```python
from build123d import *

# Parameters (mm, degrees)
SKETCH1_R           = 6
SKETCH1_R_2         = 10
BOSS_EXTRUDE5_DEPTH = 5


with BuildPart() as part:
    # Sketch1 → Boss-Extrude5 (new body)
    with BuildSketch(Plane.XY):
        with BuildLine():
            ThreePointArc((-70.058465936, -58.078352807), (-72.989066837, -63.721836205), (-74, -70))
            Line((-74, -70), (-74, -102))
            ThreePointArc((-74, -102), (-57.94255977, -121.607555239), (-35.554377754, -109.730395847))
            ThreePointArc((-35.554377754, -109.730395847), (-10.665501502, -73.723982253), (26.649375188, -50.843467428))
            ThreePointArc((26.649375188, -50.843467428), (48.384433069, -44.417618227), (70.872883052, -47.241427079))
            ThreePointArc((70.872883052, -47.241427079), (100.915737424, -45.173387051), (91.224909648, -16.661323894))
            ThreePointArc((91.224909648, -16.661323894), (58.568789172, -9.425322294), (25.12069127, -9.506995785))
            ThreePointArc((25.12069127, -9.506995785), (17.4015399, -7.087809111), (13.997757222, 0.250584822))
            ThreePointArc((13.997757222, 0.250584822), (-3.45943961, 13.565849682), (-12.408356532, -6.483262156))
            ThreePointArc((-12.408356532, -6.483262156), (-11.834915893, -14.73854087), (-17.505199272, -20.765675115))
            ThreePointArc((-17.505199272, -20.765675115), (-45.782270653, -36.604484887), (-70.058465936, -58.078352807))
        make_face()
        with BuildLine():
            ThreePointArc((-44, -102), (-54, -112), (-64, -102))
            Line((-64, -102), (-64, -70))
            ThreePointArc((-64, -70), (-54, -60), (-44, -70))
            Line((-44, -70), (-44, -102))
        make_face(mode=Mode.SUBTRACT)
        Circle(SKETCH1_R, mode=Mode.SUBTRACT)
        with Locations((85.098500813, -34.646515436)):
            Circle(SKETCH1_R_2, mode=Mode.SUBTRACT)
    extrude(amount=BOSS_EXTRUDE5_DEPTH)


solid = part.part
```
Check sheet for the modelled part. Datum: model origin and axes. Units: mm. A direction names the side the tool comes from. Round coordinates to 2 decimals unless told otherwise and drop trailing zeros. Order: outer loops, then holes, each group sorted by start corner. A loop starts at its lowest first (then second) coordinate and runs counter-clockwise, first axis right, second up. Notation, with made-up numbers: (82, 18) - (136, 18) arc R22 ccw to (136, 30) - close; hole circle Ø11 at (53, -14). An arc over 180 degrees is marked (long way). Write item = value, one per line.
Q1. Thickness scan on line 1 along X through (y, z) = (-81, 3); line 2 along X through (y, z) = (-26, 1.4); line 3 along Y through (x, z) = (86.5, 0.45). Record the ranges inside material, lowest first.
Computed:
line_1 = -74 to -64, -44 to -17.65
line_2 = -28.51 to 80.07, 90.12 to 102.02
line_3 = -53.59 to -44.55, -24.75 to -15.14
Q2. Draft check along Y on faces 1 (the face through (-6, 0, 2)), 2 (the face through (-72.96, -63.64, 2.46)), 3 (the face through (100.641, -45.575, 2.465)). Enter one of: pulls with the +Y half, pulls with the -Y half, needs draft (parallel to the pull), parting line crosses it, or undercut.
Computed:
face_1 = undercut
face_2 = pulls with the +Y half
face_3 = parting line crosses it
Q3. Tool access check on faces 4 (the face through (-54, -60, 2)), 5 (the face through (1, -44, 5)). Record the directions out of +Z, -Z, +X, -X, +Y, -Y that give a thin tool (end or side, any length) a straight path to the whole face; none if there is none.
Computed:
face_4 = +Z, -Z
face_5 = +Z, +X, -X, +Y, -Y
Q4. Section check A-A (y = -97). Record the boundary of the cut face in (x, z).
Computed:
outline = (-74, 0) - (-64, 0) - (-64, 5) - (-74, 5) - close; (-44, 0) - (-29.18, 0) - (-29.18, 5) - (-44, 5) - close
Q5. Go/stop test with flat-tipped pins: pin 1 (2 mm diameter, centred on y = -33, z = 3.5, fed in from +X); pin 2 (1.5 mm diameter, centred on y = -79.5, z = 2.5, fed in from +X); pin 3 (2 mm diameter, centred on x = 2, z = 1.5, fed in from -Y); pin 4 (6 mm diameter, centred on x = 11.5, y = -15.5, fed in from -Z). Record where each tip stops, or that it passes through.
Computed:
pin_1 = 104.09
pin_2 = -15.63
pin_3 = -64.16
pin_4 = 0
Q6. Section check B-B (x = -54). Record the boundary of the cut face in (y, z), and give its area (3 significant figures).
Computed:
outline = (-122, 0) - (-112, 0) - (-112, 5) - (-122, 5) - close; (-60, 0) - (-42.87, 0) - (-42.87, 5) - (-60, 5) - close
area = 136 mm^2
Q7. Section check C-C (z = 3.4). Record the boundary of the cut face in (x, y), and give its area (3 significant figures).
Computed:
outline = (-74, -102) arc R20 ccw to (-35.55, -109.73) arc R106 cw to (26.65, -50.84) arc R55.35 cw to (70.87, -47.24) arc R19 ccw (long way) to (91.22, -16.66) arc R152 ccw to (25.12, -9.51) arc R10 cw to (14, 0.25) arc R14 ccw (long way) to (-12.41, -6.48) arc R10.33 cw to (-17.51, -20.77) arc R152 ccw to (-70.06, -58.08) arc R20 ccw to (-74, -70) - close; hole (-64, -102) arc R10 ccw to (-44, -102) - (-44, -70) arc R10 ccw to (-64, -70) - close; hole circle Ø12 at (0, 0); hole circle Ø20 at (85.1, -34.65)
area = 8,320 mm^2
Q8. Section check D-D (x = 8). Record the boundary of the cut face in (y, z), and give its area (3 significant figures).
Computed:
outline = (-59.61, 0) - (11.49, 0) - (11.49, 5) - (-59.61, 5) - close
area = 355 mm^2
